Geometry: see drawing. Coordinates: mm, zero at the bounding-box minimum. Give positions to 0.01 mm unless a question says otherwise; leave off trailing zeros. Order: outer loops, then holes, each group sorted by start corner. A loop starts at its lowest first (then second) coordinate and runs counter-clockwise, first axis right, second up. Notation, with made-up numbers: M 83,60.25 L 91,60.25 A14 cw 91,67.25 Z; hole C 76.25,48 d3. An arc over 180 degrees is marked long. Use a Markdown table: item, result.
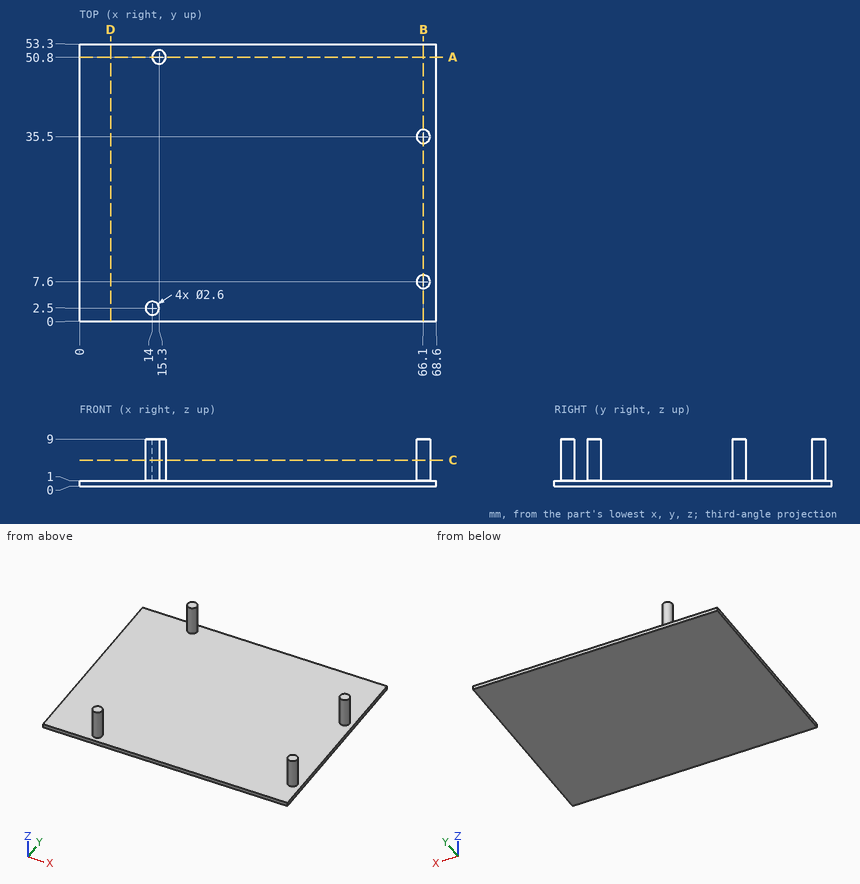
1) Cut plane A-A on y = 50.8. Return loops of the section in (x, z), and give its area (3 significant figures).
Response values:
| item | result |
|---|---|
| outline | M 0,0 L 68.6,0 L 68.6,1 L 16.6,1 L 16.6,9 L 14,9 L 14,1 L 0,1 Z |
| area | 89.4 mm² |
2) Cut plane C-C on z = 5. Return loops of the section in (x, y), and give its area (3 significant figures).
Response values:
| item | result |
|---|---|
| outline | C 14,2.5 d2.6; C 15.3,50.8 d2.6; C 66.1,7.6 d2.6; C 66.1,35.5 d2.6 |
| area | 21.2 mm² |
3) Material intervals for line 1 (Z direction, x = 45, y = 48); line 2 (X direction, y = 8.5, z = 2.5), sorted ascending. Write a range as from..to.
Response values:
| item | result |
|---|---|
| line 1 | z = 0..1 |
| line 2 | x = 65.16..67.04 |
4) Cut plane D-D on x = 6. Return loops of the section in (y, z), and give its area (3 significant figures).
Response values:
| item | result |
|---|---|
| outline | M 0,0 L 53.3,0 L 53.3,1 L 0,1 Z |
| area | 53.3 mm² |
5) Cut plane B-B on x = 66.1. Return loops of the section in (y, z), and give its area (3 significant figures).
Response values:
| item | result |
|---|---|
| outline | M 0,0 L 53.3,0 L 53.3,1 L 36.8,1 L 36.8,9 L 34.2,9 L 34.2,1 L 8.9,1 L 8.9,9 L 6.3,9 L 6.3,1 L 0,1 Z |
| area | 94.9 mm² |
